The model under review builds one solid part; all positions refer to its coordinate system, in mm. A direction names the side the tool comes from. Round coordinates to 2 decimals unless told otherwise and drop trailing zeros. Order: outer loops, then holes, each group sorted by start corner. A loop starts at its lowest first (then second) coordinate and runs counter-clockwise, first axis right, second up.
```python
from build123d import *

# Parameters (mm, degrees)
F0_R     = 1.7947651686
F1_DEPTH = 7.62
F2_R     = 2.54
F3_R     = 1.269


# Not quite as in the source:
# - a fillet or chamfer is up to 0.001 mm smaller than in the source, because OpenCascade refuses the exact size


with BuildPart() as f1:
    # F0 (on Top) → F1 (new body)
    with BuildSketch(Plane.XY):
        with BuildLine():
            ThreePointArc((-3.0625740785, 3.6819641418), (-1.865183548, 2.011379827), (-1.4421620036, 0))
            ThreePointArc((-1.4421620036, 0), (-1.4498583422, -0.2771315824), (-1.4729236329, -0.5534088705))
            Line((-1.4729236329, -0.5534088705), (4.4801407494, -0.5534088705))
            Line((4.4801407494, -0.5534088705), (4.4801407494, 3.6819641418))
            Line((4.4801407494, 3.6819641418), (-3.0625740785, 3.6819641418))
        make_face()
        with BuildLine():
            add(Edge.make_bspline(
                [(4.4801407494, 3.6819641418), (14.6919268718, 3.3504103776), (12.7431834117, -10.4070426896), (4.4801407494, -8.5037574172)],
                knots=[0, 0, 0, 0, 12.185721559, 12.185721559, 12.185721559, 12.185721559], degree=3))
            Line((4.4801407494, 3.6819641418), (4.4801407494, -0.5534088705))
            add(Edge.make_bspline(
                [(4.4801407494, -0.5534088705), (9.772202, -1.5405191807), (7.8137687942, -7.3264148086), (4.4801407494, -8.5037574172)],
                knots=[0, 0, 0, 0, 7.9503485467, 7.9503485467, 7.9503485467, 7.9503485467], degree=3))
        make_face()
        with BuildLine():
            ThreePointArc((-1.4729236329, -0.5534088705), (-1.4498583422, -0.2771315824), (-1.4421620036, 0))
            ThreePointArc((-1.4421620036, 0), (-1.865183548, 2.011379827), (-3.0625740785, 3.6819641418))
            ThreePointArc((-3.0625740785, 3.6819641418), (-11.1104438204, -1.7546257881), (-1.4729236329, -0.5534088705))
        make_face()
        with Locations((-6.4355200157, 0)):
            Circle(F0_R, mode=Mode.SUBTRACT)
    extrude(amount=F1_DEPTH)

    # F2
    f2_edges = [f1.edges().sort_by_distance(p)[0] for p in [
        (1.503609, -0.553409, 7.62),
        (7.731849, -4.321745, 7.62),
        (1.503609, -0.553409, 0),
        (7.731849, -4.321745, 0),
    ]]
    fillet(f2_edges, radius=F2_R)

    # F3 (radius 1.27 in the source; OpenCascade refuses exactly that, so slightly less here)
    f3_edges = [f1.edges().sort_by_distance(p)[0] for p in [
        (-11.110444, -1.754626, 7.62),
        (-11.110444, -1.754626, 0),
        (-8.230285, 0, 0),
        (-8.230285, 0, 7.62),
    ]]
    fillet(f3_edges, radius=F3_R)


solid = f1.part
```
(1) For faces 4 (the flat face through (1, -0.553, 4)), 5 (the flat face through (1.4, 2.3, 7.62)), list the 3-axis set-ups (+Z, -Z, +X, -X, +Y, -Y) from which the entire face can be reached by the end or side of a thin tool; tool diameter is ignored.
Data:
face 4: +Z, -Z, -Y
face 5: +Z, +X, -X, +Y, -Y
(2) To check wall thickness, follow probe 1 along X at (y, z) = (-0.5, 7); probe 2 along X at (y, z) = (-2.75, 7.25); probe 3 along Y at (x, z) = (-8, 7). State the ranges of each line that lie inside material, in increasing order.
Data:
probe 1: x = -11.22 to -8.34, -4.53 to -1.65, 6.79 to 11.04
probe 2: x = -10.15 to -2.72, 8.83 to 11.43
probe 3: y = -4.55 to -1.2, 1.2 to 4.55
(3) Draft analysis for pull direction Y (two halves, no side actions). For faces 1 (the flat face through (1, 3.682, 4)), 2 (the cylindrical face through (-4.78, -0.69, 3.77)), 3 (the flat face through (1.4, 2.3, 0)), state which applies: pulls with the +Y half, pulls with the -Y half, needs draft (parallel to the pull), parting line crosses it, or undercut.
Data:
face 1: pulls with the +Y half
face 2: undercut
face 3: needs draft
(4) Consider section A-A (x = 1.5). Write out the cut boundary in (y, z), and give its area (3 significant figures).
Data:
outline: (-0.55, 2.54) arc R2.54 ccw to (1.99, 0) - (3.68, 0) - (3.68, 7.62) - (1.99, 7.62) arc R2.54 ccw to (-0.55, 5.08) - close
area: 29.5 mm2
(5) Insertion check: pin 1 (4 mm diameter, centred on y = 0.5, z = 4, fed in from -X); pin 2 (1 mm diameter, centred on y = -5.5, z = 4, fed in from +X); pin 3 (0.8 mm diameter, centred on x = 2, z = 3.5, fed in from -Y); pin 4 (4 mm diameter, centred on x = -1, z = 4, fed in from +Y). Each pin has a flat end and moves straight along its axis. Give the tip position at first contact, or say it passes through.
Data:
pin 1: stops at x = -11.43
pin 2: stops at x = 11.04
pin 3: stops at y = -0.55
pin 4: stops at y = 3.68
